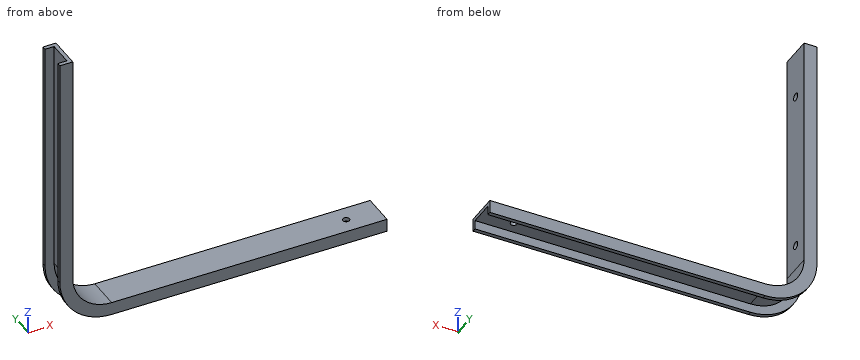
```python
from build123d import *

# Parameters (mm, degrees)
ESQUISSE1_W                  = 450
ESQUISSE1_H                  = 25
EXTRUSION1_DEPTH             = 10
PLIAGE_START                 = -12.5
PLIAGE_1_DEPTH               = 25
PLIAGE_1_2_DEPTH             = 25
ESQUISSE5_R                  = 3
ENL_V_MAT_EXTRU_1_DEPTH      = 330.361564282
ESQUISSE7_R                  = 2.5
ENL_V_MAT_EXTRU_2_DEPTH      = 331.27116136
ENL_V_MAT_EXTRU_3_DEPTH      = 9.5
ENL_V_MAT_EXTRU_3_DEPTH_BACK = 9.5


# Read off the part's stored shape, not the designer's step: Pliage 1
with BuildPart() as part:
    # Esquisse1 → Extrusion1 (new body)
    with BuildSketch(Plane.XY):
        with Locations((-225, 0)):
            Rectangle(ESQUISSE1_W, ESQUISSE1_H)
    extrude(amount=EXTRUSION1_DEPTH)

    # Pliage 1 outline → Pliage 1 (cut)
    with BuildSketch(Plane(origin=(0, 0, 0), x_dir=(1, 0, 0), z_dir=(0, 1, 0)).offset(PLIAGE_START)):
        with BuildLine():
            Line((-450, -10), (-238.968577392, -10))
            ThreePointArc((-238.968577392, -10), (-226.653199905, -2.583426132), (-212.511064281, 0))
            Line((-212.511064281, 0), (-450, 0))
            Line((-450, 0), (-450, -10))
        make_face()
    extrude(amount=PLIAGE_1_DEPTH, mode=Mode.SUBTRACT)

    # Pliage 1 2 outline → Pliage 1 2 (add)
    with BuildSketch(Plane(origin=(0, 0, 0), x_dir=(1, 0, 0), z_dir=(0, 1, 0)).offset(PLIAGE_START)):
        with BuildLine():
            ThreePointArc((-238.968577392, -10), (-248.968577392, -23.542486889), (-252.511064281, -40))
            Line((-252.511064281, -40), (-252.511064281, -222.511064281))
            Line((-252.511064281, -222.511064281), (-242.511064281, -222.511064281))
            Line((-242.511064281, -222.511064281), (-242.511064281, -40))
            ThreePointArc((-242.511064281, -40), (-233.724267717, -18.786796564), (-212.511064281, -10))
            Line((-212.511064281, -10), (-238.968577392, -10))
        make_face()
    extrude(amount=PLIAGE_1_2_DEPTH)

    # Esquisse5 → Enlèv. mat.-Extru.1 (cut, through all)
    with BuildSketch(Plane(origin=(-242.511064281, 0, 0), x_dir=(0, 0, -1), z_dir=(1, 0, 0))):
        with Locations((-185, 0)):
            Circle(ESQUISSE5_R)
        with Locations((-60, 0)):
            Circle(ESQUISSE5_R)
    extrude(amount=-ENL_V_MAT_EXTRU_1_DEPTH, mode=Mode.SUBTRACT)

    # Esquisse7 → Enlèv. mat.-Extru.2 (cut, through all)
    with BuildSketch(Plane.XY.offset(10)):
        with Locations((-25, 0)):
            Circle(ESQUISSE7_R)
    extrude(amount=-ENL_V_MAT_EXTRU_2_DEPTH, mode=Mode.SUBTRACT)

    # Esquisse8 → Enlèv. mat.-Extru.3 (cut, two sides: drawn at the far end of the back side and taken through both)
    with BuildSketch(Plane(origin=(0, 0, 0), x_dir=(1, 0, 0), z_dir=(0, 1, 0)).offset(-ENL_V_MAT_EXTRU_3_DEPTH_BACK)):
        with BuildLine():
            Line((0, -7), (-212.511064281, -7))
            ThreePointArc((-212.511064281, -7), (-235.84558806, -16.665476221), (-245.511064281, -40))
            Line((-245.511064281, -40), (-245.511064281, -222.511064281))
            Line((-245.511064281, -222.511064281), (-252.511064281, -222.511064281))
            Line((-252.511064281, -222.511064281), (-252.511064281, -40))
            ThreePointArc((-252.511064281, -40), (-240.795335529, -11.715728753), (-212.511064281, 0))
            Line((-212.511064281, 0), (0, 0))
            Line((0, 0), (0, -7))
        make_face()
    extrude(amount=ENL_V_MAT_EXTRU_3_DEPTH + ENL_V_MAT_EXTRU_3_DEPTH_BACK, mode=Mode.SUBTRACT)


solid = part.part
```
Geometry check sheet. Reference: the model listing, model coordinates, mm. Round coordinates to 2 decimals unless told otherwise and drop trailing zeros. Loops run counter-clockwise (first coordinate to the right, second up) from the corner with the lowest first, then second, coordinate; pieces in that order, holes last. Notation, with made-up numbers: (69.5, 87) - (91.5, 87) arc R8 ccw to (91.5, 94) - close; hole circle Ø2 at (-36, -18). An arc over 180 degrees is marked (long way). Write item = value, one per line. Start each with the question number.
1. Section check A-A on z = 60. Enter the section's corners in (x, y), then the cut area to 3 significant figures.
2. Section check B-B on x = -182. Enter the section's corners in (y, z).
3. Depth check by flat-ended pin: pin 1 (5 mm diameter, centred on y = 0, z = 185, fed in from -X); pin 2 (1 mm diameter, centred on x = -226.5, y = -3.5, fed in from -Z); pin 3 (12 mm diameter, centred on y = -4.5, z = 64, fed in from +X); pin 4 (5.5 mm diameter, centred on y = 2, z = 116.5, fed in from -X). Enter the tip coordinate at first touch or a pass-through.
4. Thickness scan on line 1 (Y direction, x = -25, z = 8); line 2 (Y direction, x = -244.3, z = 185); line 3 (Z direction, x = -157, y = -5.25). Record the ranges inside material, lowest first.
Working result:
q1.outline = (-252.51, -12.5) - (-242.51, -12.5) - (-242.51, -3) - (-245.51, -3) - (-245.51, -9.5) - (-252.51, -9.5) - close; (-252.51, 9.5) - (-245.51, 9.5) - (-245.51, 3) - (-242.51, 3) - (-242.51, 12.5) - (-252.51, 12.5) - close
q1.area = 99.0 mm^2
q2.outline = (-12.5, 0) - (-9.5, 0) - (-9.5, 7) - (9.5, 7) - (9.5, 0) - (12.5, 0) - (12.5, 10) - (-12.5, 10) - close
q3.pin_1 = through
q3.pin_2 = 9.88
q3.pin_3 = -242.51
q3.pin_4 = -245.51
q4.line_1 = -12.5 to -2.5, 2.5 to 12.5
q4.line_2 = -12.5 to -3, 3 to 12.5
q4.line_3 = 7 to 10
